The listing builds one solid part. Answer for the finished solid, in the listing's coordinates (mm). Face numbers are marked on the shaded views. A direction names the side the tool comes from. Round coordinates to 2 decimals unless told otherwise and drop trailing zeros. Write each loop counter-clockwise with the first axis right and the second up, starting at its lowest first coordinate (ties: lowest second). Pieces come first, ordered by that corner, then holes. Notation, with made-up numbers: (84, -22.75) - (123, -22.75) arc R21 cw to (123, 4.25) - close; hole circle Ø1 at (11.5, -39.75). An arc over 180 degrees is marked (long way). Use a Markdown table: item, result. Add a question column.
1) A cutting plane is placed at D-D (x = -10). Give the vertices of the cut face in (y, z).
2) A cutting plane is placed at B-B (y = 2.5). Give the vertices of the cut face in (x, z).
3) Each of these flat-tipped pins is pushed along its axis until it touches: P1, Ø5, axis at x = 2, z = -1, coming from the -Y side; P2, Ø4, axis at y = 20, z = -0.5, coming from the -X side; P3, Ø1.6, axis at x = 17.5, y = 8.5, coming from the -Z side; P4, Ø5, axis at x = -13.5, z = 0, coming from the +Y side. Where does it stop, or does it pass through?
4) A tool of negligible diameter and unlimited length cuts with its end or side. For the marked faces 4, 5 and 6, from which of +Z, -Z, +X, -X, +Y, -Y can it reach the whole face along a straight path? Write none if from no direction.
5) A cutting plane is placed at C-C (z = 3.5). Give the vertices of the cut face in (x, y).
6) Determine the mould class of the marked faces 1, 2 and 3 for opening direction X: +X half, -X half, draft (parallel to the pull), parting line (faces both ways), or undercut.
7) Find the intervals of material crossed by probe 1 along X at (y, z) = (16, -1.75); probe 2 along Y at (x, z) = (-14, 0.25); probe 3 along X at (y, z) = (10.25, 3), in increasing order. Write a range as from..to.
8) A cutting plane is placed at A-A (y = 10.75). Give the vertices of the cut face in (x, z).
```python
from build123d import *

# Parameters (mm, degrees)
BOSS_EXTRUDE1_DEPTH = 3
SKETCH2_W           = 3
SKETCH2_H           = 10
BOSS_EXTRUDE2_DEPTH = 14
SKETCH3_W           = 1.5
SKETCH3_H           = 5
BOSS_EXTRUDE3_DEPTH = 27


with BuildPart() as part:
    # Sketch1 → Boss-Extrude1 (new body)
    with BuildSketch(Plane(origin=(0, 0, 0), x_dir=(1, 0, 0), z_dir=(0, 1, 0))):
        Polygon((18, 2.5), (16.5, 2.5), (-15, 5), (-18, 5), (-18, -5), (-15, -5), (16.5, -2.5), (18, -2.5), align=None)
    extrude(amount=BOSS_EXTRUDE1_DEPTH)

    # Sketch2 → Boss-Extrude2 (add)
    with BuildSketch(Plane(origin=(0, 3, 0), x_dir=(1, 0, 0), z_dir=(0, 1, 0))):
        with Locations((-16.5, 0)):
            Rectangle(SKETCH2_W, SKETCH2_H)
    extrude(amount=BOSS_EXTRUDE2_DEPTH)

    # Sketch3 → Boss-Extrude3 (add)
    with BuildSketch(Plane(origin=(0, 3, 0), x_dir=(1, 0, 0), z_dir=(0, 1, 0))):
        with Locations((17.25, 0)):
            Rectangle(SKETCH3_W, SKETCH3_H)
    extrude(amount=BOSS_EXTRUDE3_DEPTH)


solid = part.part
```
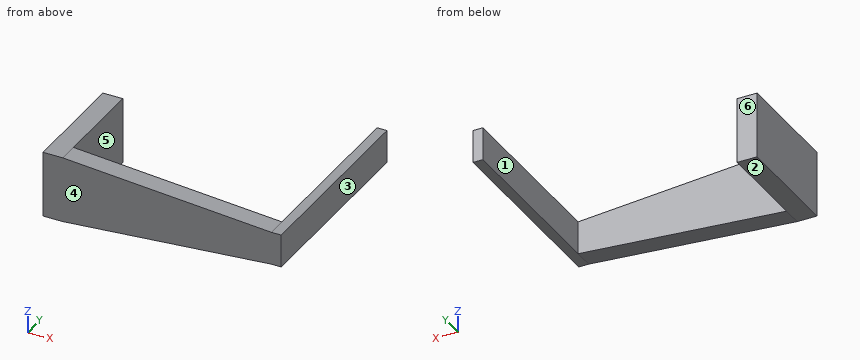
Entries:
| question | item | result |
|---|---|---|
| 1 | outline | (0, -4.6) - (3, -4.6) - (3, 4.6) - (0, 4.6) - close |
| 2 | outline | (-18, -5) - (-15, -5) - (16.5, -2.5) - (18, -2.5) - (18, 2.5) - (16.5, 2.5) - (-15, 5) - (-18, 5) - close |
| 3 | P1 | stops at y = 0 |
| 3 | P2 | stops at x = 16.5 |
| 3 | P3 | stops at z = -2.5 |
| 3 | P4 | stops at y = 17 |
| 4 | face 4 | +Z, -Z, +X, -X, -Y |
| 4 | face 5 | +Z, -Z, +Y |
| 4 | face 6 | +Z, -Z, -X, +Y |
| 5 | outline | (-18, 0) - (3.9, 0) - (3.9, 3) - (-15, 3) - (-15, 17) - (-18, 17) - close |
| 6 | face 1 | undercut |
| 6 | face 2 | draft |
| 6 | face 3 | +X half |
| 7 | probe 1 | x = -18..-15, 16.5..18 |
| 7 | probe 2 | y = 0..3 |
| 7 | probe 3 | x = -18..-15 |
| 8 | outline | (-18, -5) - (-15, -5) - (-15, 5) - (-18, 5) - close; (16.5, -2.5) - (18, -2.5) - (18, 2.5) - (16.5, 2.5) - close |
